Check sheet for the modelled part. Datum: model origin and axes. Units: mm. A direction names the side the tool comes from. Give positions to 0.01 mm unless a question says otherwise; leave off trailing zeros. Loops run counter-clockwise (first coordinate to the right, second up) from the corner with the lowest first, then second, coordinate; pieces in that order, holes last. Notation, with made-up numbers: (71, 10.5) -> (96, 10.5) arc R22 cw to (96, 31.5) -> close; hole circle Ø10 at (29.5, 63). An arc over 180 degrees is marked (long way). Answer as CSV lines item,"result". Start each with the question number.
(1) Release check for a two-part mould opening along Y. For faces 1 (the face through (2, 79, 50)), 2 (the face through (2, 49, 100)) record: pulls with the +Y half, pulls with the -Y half, needs draft (parallel to the pull), parting line crosses it, or undercut.
(2) Access from +Z, -Z, +X, -X, +Y, -Y to the whole of each face (thin tool, end or side, straight path). Record for faces 3 (the face through (2, 50, 42.5)), 4 (the face through (0, 51, 51)).
(3) Section check C-C on y = 92. Enter the section's corners in (x, z), plus the area to 3 significant figures.
(4) Section check A-A on z = 73. Enter the section's corners in (x, y), plus the area to 3 significant figures.
(5) Gauge pin test, flat ends, axial feed: pin 1 Ø4.5 at (y, z) = (8, 9) entering from +X; pin 2 Ø3 at (y, z) = (8, 73) entering from +X. Record the tip position at first contact, or that the pin passes through.
(6) Section check D-D on x = 2.4. State how many separate pieces and enclosed holes the cut face has, plus the area to 3 significant figures.
(7) Material ranges on line 1 (Y direction, x = 1.75, z = 27); line 2 (Z direction, x = 3.25, y = 72.5); line 3 (Z direction, x = 4.5, y = 69.5), recorded low to high. Write a range as from..to.
(8) Section check B-B on y = 56. Enter the section's corners in (x, z).
from build123d import *

# Parameters (mm, degrees)
SKETCH_1_W      = 100
SKETCH_1_H      = 100
SKETCH_1_R      = 2
SKETCH_1_W_2    = 5
SKETCH_1_H_2    = 15
SKETCH_1_W_3    = 10
SKETCH_1_H_3    = 5
EXTRUDE_1_DEPTH = 5


with BuildPart() as part:
    # 草图1 → 凸台-拉伸1 (new body)
    with BuildSketch(Plane(origin=(0, 0, 0), x_dir=(0, 0, -1), z_dir=(1, 0, 0))):
        with Locations((-50, 50)):
            Rectangle(SKETCH_1_W, SKETCH_1_H)
        with Locations((-91, 92)):
            Circle(SKETCH_1_R, mode=Mode.SUBTRACT)
        with Locations((-27, 92)):
            Circle(SKETCH_1_R, mode=Mode.SUBTRACT)
        with Locations((-91, 8)):
            Circle(SKETCH_1_R, mode=Mode.SUBTRACT)
        with Locations((-27, 8)):
            Circle(SKETCH_1_R, mode=Mode.SUBTRACT)
        with Locations((-73, 92)):
            Circle(SKETCH_1_R, mode=Mode.SUBTRACT)
        with Locations((-73, 68)):
            Circle(SKETCH_1_R, mode=Mode.SUBTRACT)
        with Locations((-91, 68)):
            Circle(SKETCH_1_R, mode=Mode.SUBTRACT)
        with Locations((-9, 92)):
            Circle(SKETCH_1_R, mode=Mode.SUBTRACT)
        with Locations((-9, 68)):
            Circle(SKETCH_1_R, mode=Mode.SUBTRACT)
        with Locations((-27, 68)):
            Circle(SKETCH_1_R, mode=Mode.SUBTRACT)
        with Locations((-73, 8)):
            Circle(SKETCH_1_R, mode=Mode.SUBTRACT)
        with Locations((-73, 32)):
            Circle(SKETCH_1_R, mode=Mode.SUBTRACT)
        with Locations((-91, 32)):
            Circle(SKETCH_1_R, mode=Mode.SUBTRACT)
        with Locations((-9, 8)):
            Circle(SKETCH_1_R, mode=Mode.SUBTRACT)
        with Locations((-9, 32)):
            Circle(SKETCH_1_R, mode=Mode.SUBTRACT)
        with Locations((-27, 32)):
            Circle(SKETCH_1_R, mode=Mode.SUBTRACT)
        with Locations((-60, 50)):
            Rectangle(SKETCH_1_W_2, SKETCH_1_H_2, mode=Mode.SUBTRACT)
        with Locations((-40, 50)):
            Rectangle(SKETCH_1_W_2, SKETCH_1_H_2, mode=Mode.SUBTRACT)
        with Locations((-50, 37.5)):
            Rectangle(SKETCH_1_W_3, SKETCH_1_H_3, mode=Mode.SUBTRACT)
        with Locations((-50, 62.5)):
            Rectangle(SKETCH_1_W_3, SKETCH_1_H_3, mode=Mode.SUBTRACT)
        with BuildLine():
            Line((-36, 74), (-64, 74))
            ThreePointArc((-64, 74), (-64.707106781, 73.707106781), (-65, 73))
            Line((-65, 73), (-65, 72))
            ThreePointArc((-65, 72), (-64.707106781, 71.292893219), (-64, 71))
            Line((-64, 71), (-36, 71))
            ThreePointArc((-36, 71), (-35.292893219, 71.292893219), (-35, 72))
            Line((-35, 72), (-35, 73))
            ThreePointArc((-35, 73), (-35.292893219, 73.707106781), (-36, 74))
        make_face(mode=Mode.SUBTRACT)
        with BuildLine():
            Line((-36, 82), (-64, 82))
            ThreePointArc((-64, 82), (-64.707106781, 81.707106781), (-65, 81))
            Line((-65, 81), (-65, 80))
            ThreePointArc((-65, 80), (-64.707106781, 79.292893219), (-64, 79))
            Line((-64, 79), (-36, 79))
            ThreePointArc((-36, 79), (-35.292893219, 79.292893219), (-35, 80))
            Line((-35, 80), (-35, 81))
            ThreePointArc((-35, 81), (-35.292893219, 81.707106781), (-36, 82))
        make_face(mode=Mode.SUBTRACT)
        with BuildLine():
            Line((-36, 90), (-64, 90))
            ThreePointArc((-64, 90), (-64.707106781, 89.707106781), (-65, 89))
            Line((-65, 89), (-65, 88))
            ThreePointArc((-65, 88), (-64.707106781, 87.292893219), (-64, 87))
            Line((-64, 87), (-36, 87))
            ThreePointArc((-36, 87), (-35.292893219, 87.292893219), (-35, 88))
            Line((-35, 88), (-35, 89))
            ThreePointArc((-35, 89), (-35.292893219, 89.707106781), (-36, 90))
        make_face(mode=Mode.SUBTRACT)
        with BuildLine():
            Line((-36, 29), (-64, 29))
            ThreePointArc((-64, 29), (-64.707106781, 28.707106781), (-65, 28))
            Line((-65, 28), (-65, 27))
            ThreePointArc((-65, 27), (-64.707106781, 26.292893219), (-64, 26))
            Line((-64, 26), (-36, 26))
            ThreePointArc((-36, 26), (-35.292893219, 26.292893219), (-35, 27))
            Line((-35, 27), (-35, 28))
            ThreePointArc((-35, 28), (-35.292893219, 28.707106781), (-36, 29))
        make_face(mode=Mode.SUBTRACT)
        with BuildLine():
            Line((-36, 21), (-64, 21))
            ThreePointArc((-64, 21), (-64.707106781, 20.707106781), (-65, 20))
            Line((-65, 20), (-65, 19))
            ThreePointArc((-65, 19), (-64.707106781, 18.292893219), (-64, 18))
            Line((-64, 18), (-36, 18))
            ThreePointArc((-36, 18), (-35.292893219, 18.292893219), (-35, 19))
            Line((-35, 19), (-35, 20))
            ThreePointArc((-35, 20), (-35.292893219, 20.707106781), (-36, 21))
        make_face(mode=Mode.SUBTRACT)
        with BuildLine():
            Line((-36, 13), (-64, 13))
            ThreePointArc((-64, 13), (-64.707106781, 12.707106781), (-65, 12))
            Line((-65, 12), (-65, 11))
            ThreePointArc((-65, 11), (-64.707106781, 10.292893219), (-64, 10))
            Line((-64, 10), (-36, 10))
            ThreePointArc((-36, 10), (-35.292893219, 10.292893219), (-35, 11))
            Line((-35, 11), (-35, 12))
            ThreePointArc((-35, 12), (-35.292893219, 12.707106781), (-36, 13))
        make_face(mode=Mode.SUBTRACT)
        with BuildLine():
            Line((-20, 60), (-19, 60))
            ThreePointArc((-19, 60), (-18.292893219, 59.707106781), (-18, 59))
            Line((-18, 59), (-18, 41))
            ThreePointArc((-18, 41), (-18.292893219, 40.292893219), (-19, 40))
            Line((-19, 40), (-20, 40))
            ThreePointArc((-20, 40), (-20.707106781, 40.292893219), (-21, 41))
            Line((-21, 41), (-21, 59))
            ThreePointArc((-21, 59), (-20.707106781, 59.707106781), (-20, 60))
        make_face(mode=Mode.SUBTRACT)
        with BuildLine():
            Line((-12, 60), (-11, 60))
            ThreePointArc((-11, 60), (-10.292893219, 59.707106781), (-10, 59))
            Line((-10, 59), (-10, 41))
            ThreePointArc((-10, 41), (-10.292893219, 40.292893219), (-11, 40))
            Line((-11, 40), (-12, 40))
            ThreePointArc((-12, 40), (-12.707106781, 40.292893219), (-13, 41))
            Line((-13, 41), (-13, 59))
            ThreePointArc((-13, 59), (-12.707106781, 59.707106781), (-12, 60))
        make_face(mode=Mode.SUBTRACT)
        with BuildLine():
            Line((-80, 60), (-81, 60))
            ThreePointArc((-81, 60), (-81.707106781, 59.707106781), (-82, 59))
            Line((-82, 59), (-82, 41))
            ThreePointArc((-82, 41), (-81.707106781, 40.292893219), (-81, 40))
            Line((-81, 40), (-80, 40))
            ThreePointArc((-80, 40), (-79.292893219, 40.292893219), (-79, 41))
            Line((-79, 41), (-79, 59))
            ThreePointArc((-79, 59), (-79.292893219, 59.707106781), (-80, 60))
        make_face(mode=Mode.SUBTRACT)
        with BuildLine():
            Line((-88, 60), (-89, 60))
            ThreePointArc((-89, 60), (-89.707106781, 59.707106781), (-90, 59))
            Line((-90, 59), (-90, 41))
            ThreePointArc((-90, 41), (-89.707106781, 40.292893219), (-89, 40))
            Line((-89, 40), (-88, 40))
            ThreePointArc((-88, 40), (-87.292893219, 40.292893219), (-87, 41))
            Line((-87, 41), (-87, 59))
            ThreePointArc((-87, 59), (-87.292893219, 59.707106781), (-88, 60))
        make_face(mode=Mode.SUBTRACT)
    extrude(amount=EXTRUDE_1_DEPTH)


solid = part.part
Working result:
1,face 1,"undercut"
1,face 2,"needs draft"
2,face 3,"+X, -X"
2,face 4,"+Z, -Z, -X, +Y, -Y"
3,outline,"(0, 0) -> (5, 0) -> (5, 7) -> (0, 7) -> close; (0, 11) -> (5, 11) -> (5, 25) -> (0, 25) -> close; (0, 29) -> (5, 29) -> (5, 71) -> (0, 71) -> close; (0, 75) -> (5, 75) -> (5, 89) -> (0, 89) -> close; (0, 93) -> (5, 93) -> (5, 100) -> (0, 100) -> close"
3,area,"420 mm^2"
4,outline,"(0, 0) -> (5, 0) -> (5, 6) -> (0, 6) -> close; (0, 10) -> (5, 10) -> (5, 30) -> (0, 30) -> close; (0, 34) -> (5, 34) -> (5, 66) -> (0, 66) -> close; (0, 70) -> (5, 70) -> (5, 90) -> (0, 90) -> close; (0, 94) -> (5, 94) -> (5, 100) -> (0, 100) -> close"
4,area,"420 mm^2"
5,pin 1,"stops at x = 5"
5,pin 2,"passes through"
6,separate pieces,"1"
6,enclosed holes,"30"
6,area,"8,780 mm^2"
7,line 1,"y = 0..6, 10..30, 34..66, 70..90, 94..100"
7,line 2,"z = 0..35, 65..100"
7,line 3,"z = 0..7.68, 10.32..25.68, 28.32..71.68, 74.32..89.68, 92.32..100"
8,outline,"(0, 0) -> (5, 0) -> (5, 10) -> (0, 10) -> close; (0, 13) -> (5, 13) -> (5, 18) -> (0, 18) -> close; (0, 21) -> (5, 21) -> (5, 37.5) -> (0, 37.5) -> close; (0, 42.5) -> (5, 42.5) -> (5, 57.5) -> (0, 57.5) -> close; (0, 62.5) -> (5, 62.5) -> (5, 79) -> (0, 79) -> close; (0, 82) -> (5, 82) -> (5, 87) -> (0, 87) -> close; (0, 90) -> (5, 90) -> (5, 100) -> (0, 100) -> close"
